Input: part model. Units: mm. Frame: model coordinates. A direction names the side the tool comes from. Round coordinates to 2 decimals unless told otherwise and drop trailing zeros. Order: outer loops, then holes, each group sorted by start corner. A loop starts at its lowest first (then second) coordinate and runs counter-clockwise, first axis right, second up. Notation, with made-up numbers: M -40,2 L 3,2 A25 cw 3,15 Z; hole C -10,-30 d1. An arc over 180 degrees is marked long. One line per question, with ' | ' between items.
```python
from build123d import *

# Parameters (mm, degrees)
SKETCH_1_R      = 1.5
EXTRUDE_1_DEPTH = 3


with BuildPart() as part:
    # 草图1 → 凸台-拉伸1 (new body)
    with BuildSketch(Plane(origin=(0, 0, 0), x_dir=(1, 0, 0), z_dir=(0, 1, 0))):
        with BuildLine():
            Line((-45, 50), (45, 50))
            ThreePointArc((45, 50), (48.535533906, 48.535533906), (50, 45))
            Line((50, 45), (50, -45))
            ThreePointArc((50, -45), (48.535533906, -48.535533906), (45, -50))
            Line((45, -50), (-45, -50))
            ThreePointArc((-45, -50), (-48.535533906, -48.535533906), (-50, -45))
            Line((-50, -45), (-50, 45))
            ThreePointArc((-50, 45), (-48.535533906, 48.535533906), (-45, 50))
        make_face()
        with Locations(Location((-45, 45, 0), (0, 0, 270))):
            Circle(SKETCH_1_R, mode=Mode.SUBTRACT)
        with Locations(Location((45, 45, 0), (0, 0, 270))):
            Circle(SKETCH_1_R, mode=Mode.SUBTRACT)
        with Locations(Location((-45, -45, 0), (0, 0, 270))):
            Circle(SKETCH_1_R, mode=Mode.SUBTRACT)
        with Locations(Location((45, -45, 0), (0, 0, 270))):
            Circle(SKETCH_1_R, mode=Mode.SUBTRACT)
        with Locations(Location((6.345, 0, 0), (0, 0, 270))):
            Circle(SKETCH_1_R, mode=Mode.SUBTRACT)
        with Locations(Location((-22.545, 0, 0), (0, 0, 270))):
            Circle(SKETCH_1_R, mode=Mode.SUBTRACT)
        with BuildLine():
            Line((-17.4, 6.2), (1.2, 6.2))
            ThreePointArc((1.2, 6.2), (2.614213562, 5.614213562), (3.2, 4.2))
            Line((3.2, 4.2), (3.2, -4.2))
            ThreePointArc((3.2, -4.2), (2.614213562, -5.614213562), (1.2, -6.2))
            Line((1.2, -6.2), (-17.4, -6.2))
            ThreePointArc((-17.4, -6.2), (-18.814213562, -5.614213562), (-19.4, -4.2))
            Line((-19.4, -4.2), (-19.4, 4.2))
            ThreePointArc((-19.4, 4.2), (-18.814213562, 5.614213562), (-17.4, 6.2))
        make_face(mode=Mode.SUBTRACT)
    extrude(amount=EXTRUDE_1_DEPTH)


solid = part.part
```
Item 1: Access query for faces 1 (the flat face through (-8, 1, 6.2)), 2 (the flat face through (-1, 1, -50)). Directions: +Z, -Z, +X, -X, +Y, -Y. A direction counts if a zero-diameter tool reaches every point of the face in a straight line with its end or side. Return the directions, or none.
Report:
face 1: +Y, -Y | face 2: -Z, +X, -X, +Y, -Y
Item 2: Section query C-C, the plane y = 1.8. Return loops of the section in (x, z) (3 decimals), plus the area to 3 significant figures.
Report:
outline: M -50,-45 A5 ccw -45,-50 L 45,-50 A5 ccw 50,-45 L 50,45 A5 ccw 45,50 L -45,50 A5 ccw -50,45 Z; hole C -45,-45 d3; hole C -45,45 d3; hole C -22.545,0 d3; hole M -19.4,-4.2 A2 ccw -17.4,-6.2 L 1.2,-6.2 A2 ccw 3.2,-4.2 L 3.2,4.2 A2 ccw 1.2,6.2 L -17.4,6.2 A2 ccw -19.4,4.2 Z; hole C 6.345,0 d3; hole C 45,-45 d3; hole C 45,45 d3 | area: 9,660 mm²
Item 3: Section query A-A, the plane z = 0. Return loops of the section in (x, y) (3 decimals), plus the area to 3 significant figures.
Report:
outline: M -50,0 L -24.045,0 L -24.045,3 L -50,3 Z; M -21.045,0 L -19.4,0 L -19.4,3 L -21.045,3 Z; M 3.2,0 L 4.845,0 L 4.845,3 L 3.2,3 Z; M 7.845,0 L 50,0 L 50,3 L 7.845,3 Z | area: 214 mm²
Item 4: Section query B-B, the plane x = -3. Return loops of the section in (y, z), plus the area to 3 significant figures.
Report:
outline: M 0,-50 L 3,-50 L 3,-6.2 L 0,-6.2 Z; M 0,6.2 L 3,6.2 L 3,50 L 0,50 Z | area: 263 mm²
Item 5: Mould query, pull axis X, two halves, no side actions, for faces 3 (the cylindrical face through (48, 1, -49)), 4 (the flat face through (1, 3, 10)), 5 (the flat face through (-8, 1, -6.2)). Classes: +X half, -X half, draft (parallel to the pull), parting line (faces both ways), or undercut.
Report:
face 3: +X half | face 4: draft | face 5: undercut
Item 6: Line query: line 1 along X through (y, z) = (1.5, 0) (3 decimals); line 2 along X through (y, z) = (2.1, -45); line 3 along X through (y, z) = (2.7, -2). Output: solid intervals per line, ascending. Write a range as from..to.
Report:
line 1: -50..-24.045, -21.045..-19.4, 3.2..4.845, 7.845..50 | line 2: -50..-46.5, -43.5..43.5, 46.5..50 | line 3: -50..-19.4, 3.2..50
